Verification items for the finished model (mm, model axes). Face numbers are marked on the shaded views. Coordinates: 2 decimals unless noted, no trailing zeros. Loops run counter-clockwise (first coordinate to the right, second up) from the corner with the lowest first, then second, coordinate; pieces in that order, holes last. Notation, with made-up numbers: M 83.5,-14.75 L 101.5,-14.75 A13 cw 101.5,3.25 Z; hole C 87,-4 d11. An arc over 180 degrees is marked long. Write item = value, one per line. Start each with the question number.
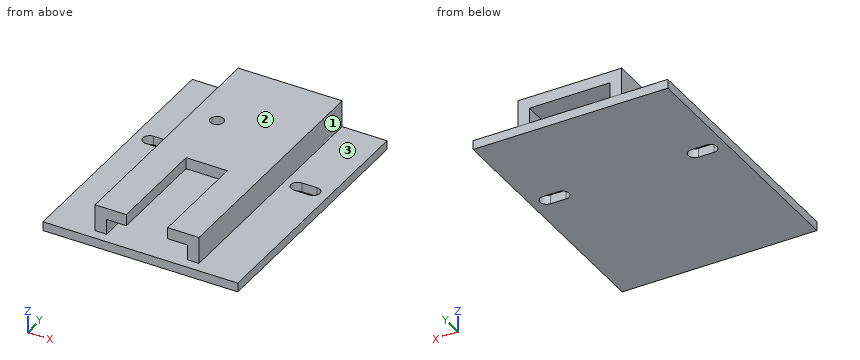
```python
from build123d import *

# Parameters (mm, degrees)
F0_W      = 75
F0_H      = 100
F1_DEPTH  = 3.5
F3_DEPTH  = 3.5
F4_W      = 40
F4_H      = 40.000004
F5_DEPTH  = 10.3
F7_DEPTH  = 40
F9_R      = 2.5
F10_DEPTH = 5.5
F11_W     = 40
F11_H     = 10.3
F12_DEPTH = 16
F8_W      = 31.1
F8_H      = 5.9
F13_DEPTH = 56.000004


with BuildPart() as f1:
    # F0 (on Top) → F1 (new body)
    with BuildSketch(Plane.XY):
        Rectangle(F0_W, F0_H)
    extrude(amount=F1_DEPTH)

    # F2 (on face) → F3 (cut, through all)
    with BuildSketch(Plane.XY.offset(3.5)):
        with BuildLine():
            Line((25.5, 8.45), (31.5, 8.45))
            ThreePointArc((31.5, 8.45), (34.05, 11.001591), (31.496817, 13.549998))
            Line((31.496817, 13.549998), (25.692115, 13.542753))
            ThreePointArc((25.692115, 13.542753), (22.951812, 11.096126), (25.5, 8.45))
        make_face()
        with BuildLine():
            ThreePointArc((-25.5, 8.45), (-22.951812, 11.096126), (-25.692115, 13.542753))
            Line((-25.692115, 13.542753), (-31.496817, 13.549998))
            ThreePointArc((-31.496817, 13.549998), (-34.05, 11.001591), (-31.5, 8.45))
            Line((-31.5, 8.45), (-25.5, 8.45))
        make_face()
    extrude(amount=-F3_DEPTH, mode=Mode.SUBTRACT)

    # F4 (on face) → F5 (join)
    with BuildSketch(Plane.XY.offset(3.5)):
        with Locations((0.25, 14.000002)):
            Rectangle(F4_W, F4_H)
    extrude(amount=F5_DEPTH)

    # F6 (on face) → F7 (join)
    with BuildSketch(Plane.XZ.offset(6)):
        Polygon((-7.71, 13.8), (-19.75, 13.8), (-19.75, 3.5), (-15.3, 3.5), (-15.3, 9.4), (-7.71, 9.4), align=None)
        Polygon((20.25, 3.5), (20.25, 13.8), (8.21, 13.8), (8.21, 9.4), (15.8, 9.4), (15.8, 3.5), align=None)
    extrude(amount=F7_DEPTH)

    # F9 (on face) → F10 (cut)
    with BuildSketch(Plane.XY.offset(13.8)):
        with Locations((-10.025, 18.8)):
            Circle(F9_R)
    extrude(amount=-F10_DEPTH, mode=Mode.SUBTRACT)

    # F11 (on face) → F12 (join)
    with BuildSketch(Plane(origin=(0, 34.000004, 0), x_dir=(-1, 0, 0), z_dir=(0, 1, 0))):
        with Locations((-0.25, 8.65)):
            Rectangle(F11_W, F11_H)
    extrude(amount=F12_DEPTH)

    # F8 (on face) → F13 (cut, through all)
    with BuildSketch(Plane.XZ.offset(6)):
        with Locations((0.25, 6.45)):
            Rectangle(F8_W, F8_H)
    extrude(amount=-F13_DEPTH, mode=Mode.SUBTRACT)


solid = f1.part
```
Q1. Sectioned sample at B-B on x = 0.5. Record the cut outline in (y, z), plus the area to 3 significant figures.
Q2. Sectioned sample at D-D on y = -35. Record the cut outline in (x, z), plus the area to 3 significant figures.
Q3. Sectioned sample at C-C on z = 7.25. Record the cut outline in (x, y), plus the area to 3 significant figures.
Q4. Gauge pin test, flat ends, axial feed: pin 1 (3.5 mm diameter, centred on x = -2, z = 11, fed in from -Y); pin 2 (8 mm diameter, centred on y = 21.5, z = 8.5, fed in from +X); pin 3 (8 mm diameter, centred on x = 16, z = 8, fed in from -Y). Record the tip position at first contact, or that the pin passes through.
Q5. Mould release check, pull along X, two halves, no side actions. Record for the marked faces 1, 2 and 3: +X half, -X half, draft (parallel to the pull), parting line (faces both ways), or undercut.
Q6. Scan lines: L1, parallel to Z at x = -12.5, y = 17; L2, parallel to X at y = -42, z = 11; L3, parallel to X at y = 11, z = 5.25. Record each from-to range of solid material in increasing order. Write a range as [from, to].
Q7. Sectioned sample at A-A on y = 11. Record the cut outline in (x, z), plus the area to 3 significant figures.
Solutions:
q1.outline = M -50,0 L 50,0 L 50,3.5 L -50,3.5 Z; M -6,9.4 L 50,9.4 L 50,13.8 L -6,13.8 Z
q1.area = 596 mm²
q2.outline = M -37.5,0 L 37.5,0 L 37.5,3.5 L 20.25,3.5 L 20.25,13.8 L 8.21,13.8 L 8.21,9.4 L 15.8,9.4 L 15.8,3.5 L -15.3,3.5 L -15.3,9.4 L -7.71,9.4 L -7.71,13.8 L -19.75,13.8 L -19.75,3.5 L -37.5,3.5 Z
q2.area = 421 mm²
q3.outline = M -19.75,-46 L -15.3,-46 L -15.3,50 L -19.75,50 Z; M 15.8,-46 L 20.25,-46 L 20.25,50 L 15.8,50 Z
q3.area = 854 mm²
q4.pin_1 = -6
q4.pin_2 = 20.25
q4.pin_3 = -46
q5.face_1 = +X half
q5.face_2 = draft
q5.face_3 = undercut
q6.L1 = [0, 3.5], [9.4, 13.8]
q6.L2 = [-19.75, -7.71], [8.21, 20.25]
q6.L3 = [-19.75, -15.3], [15.8, 20.25]
q7.outline = M -37.5,0 L -34.05,0 L -34.05,3.5 L -37.5,3.5 Z; M -22.95,0 L 22.95,0 L 22.95,3.5 L 20.25,3.5 L 20.25,13.8 L -19.75,13.8 L -19.75,3.5 L -22.95,3.5 Z; M 34.05,0 L 37.5,0 L 37.5,3.5 L 34.05,3.5 Z; hole M -15.3,3.5 L 15.8,3.5 L 15.8,9.4 L -15.3,9.4 Z
q7.area = 413 mm²
